Check sheet for the modelled part. Datum: model origin and axes. Units: mm. Round coordinates to 2 decimals unless told otherwise and drop trailing zeros. Write each loop counter-clockwise with the first axis right and the second up, starting at its lowest first coordinate (ties: lowest second). Pieces come first, ordered by that corner, then holes. Notation, with made-up numbers: (66.25, 32) - (98.25, 32) arc R24 ccw to (98.25, 47) - close; hole circle Ø11 at (31, -3.5). An arc over 180 degrees is marked (long way). Use one line per item in the form item = value. Start each with the question number.
1) Section check D-D (z = -32). Record the boundary of the cut face in (x, y).
2) Gauge pin test, flat ends, axial feed: P1, Ø4, axis at x = 15.5, y = 15.5, coming from the -Z side; P2, Ø2.5, axis at x = 15.5, y = -15.5, coming from the -Z side; P3, Ø2, axis at y = -1, z = -21, coming from the -X side; P4, Ø8, axis at x = 10, z = -90.5, coming from the -Y side. Record the tip position at first contact, or that the pin passes through.
3) Scan lines: probe 1 along Y at (x, z) = (15.5, 2.5); probe 2 along X at (y, z) = (15, 2). Record each from-to range of solid material in increasing order.
4) Section check B-B (y = 0). Record the boundary of the cut face in (x, z).
5) Section check A-A (z = 13). Record the boundary of the cut face in (x, y).
Solid Edge part; units mm, degrees
sketch "Sketch1" plane through (0, 0, 0) normal (0, 0, 1) x (1, 0, 0)
  line L0 (21.15, -21.15) -> (21.15, 21.15)
  line L1 (21.15, 21.15) -> (-21.15, 21.15)
  line L2 (-21.15, 21.15) -> (-21.15, -21.15)
  line L3 (-21.15, -21.15) -> (21.15, -21.15)
extrude "Protrusion1" add sketch "Sketch1" along normal blind 40
sketch "Sketch2" plane through (0, 0, 0) normal (0, 0, 1) x (1, 0, 0)
  circle A0 centre (0, 0) radius 11
extrude "ExtrudedProtrusion_2" add sketch "Sketch2" against normal blind 2
sketch "Sketch3" plane through (0, 0, 0) normal (0, 0, 1) x (1, 0, 0)
  circle A0 centre (0, 0) radius 4
extrude "ExtrudedProtrusion_3" add sketch "Sketch3" against normal blind 300
sketch "Sketch4" plane through (0, 0, 0) normal (0, 0, 1) x (1, 0, 0)
  circle A0 centre (15.5, 15.5) radius 1.5
  circle A1 centre (-15.5, 15.5) radius 1.5
  circle A2 centre (-15.5, -15.5) radius 1.5
  circle A3 centre (15.5, -15.5) radius 1.5
extrude "ExtrudedCutout_1" cut sketch "Sketch4" along normal blind 4.5
chamfer "Chamfer_1" distance 5 angle 45 4 edges at (21.15, 21.15, 20) (-21.15, 21.15, 20) (-21.15, -21.15, 20) (21.15, -21.15, 20)
fillet "Round_1" radius 1 8 edges at (0, 21.15, 40) (-18.65, 18.65, 40) (-21.15, 0, 40) (-18.65, -18.65, 40) (0, -21.15, 40) (18.65, -18.65, 40) (21.15, 0, 40) (18.65, 18.65, 40)
chamfer "Chamfer_2" distance 0.5 angle 45 1 edges at (-4, 0, -300)
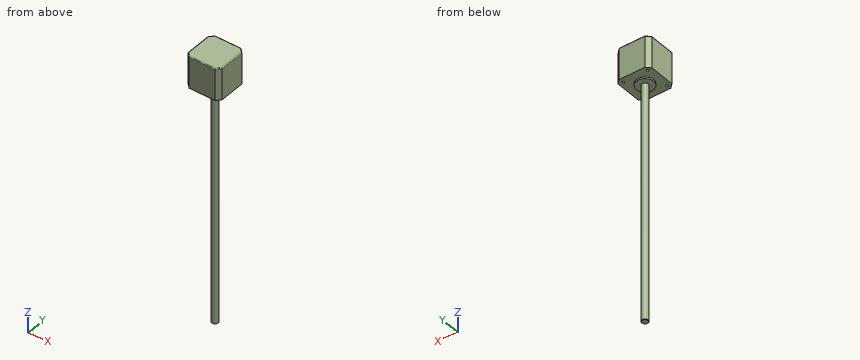
Results are:
q1.outline = circle Ø8 at (0, 0)
q2.P1 = 0
q2.P2 = 4.5
q2.P3 = -4
q2.P4 = through
q3.probe_1 = -21.15 to -17, -14 to 14, 17 to 21.15
q3.probe_2 = -21.15 to -16.91, -14.09 to 14.09, 16.91 to 21.15
q4.outline = (-21.15, 0) - (-11, 0) - (-11, -2) - (-4, -2) - (-4, -299.5) - (-3.5, -300) - (3.5, -300) - (4, -299.5) - (4, -2) - (11, -2) - (11, 0) - (21.15, 0) - (21.15, 39) arc R1 ccw to (20.15, 40) - (-20.15, 40) arc R1 ccw to (-21.15, 39) - close
q5.outline = (-21.15, -16.15) - (-16.15, -21.15) - (16.15, -21.15) - (21.15, -16.15) - (21.15, 16.15) - (16.15, 21.15) - (-16.15, 21.15) - (-21.15, 16.15) - close
